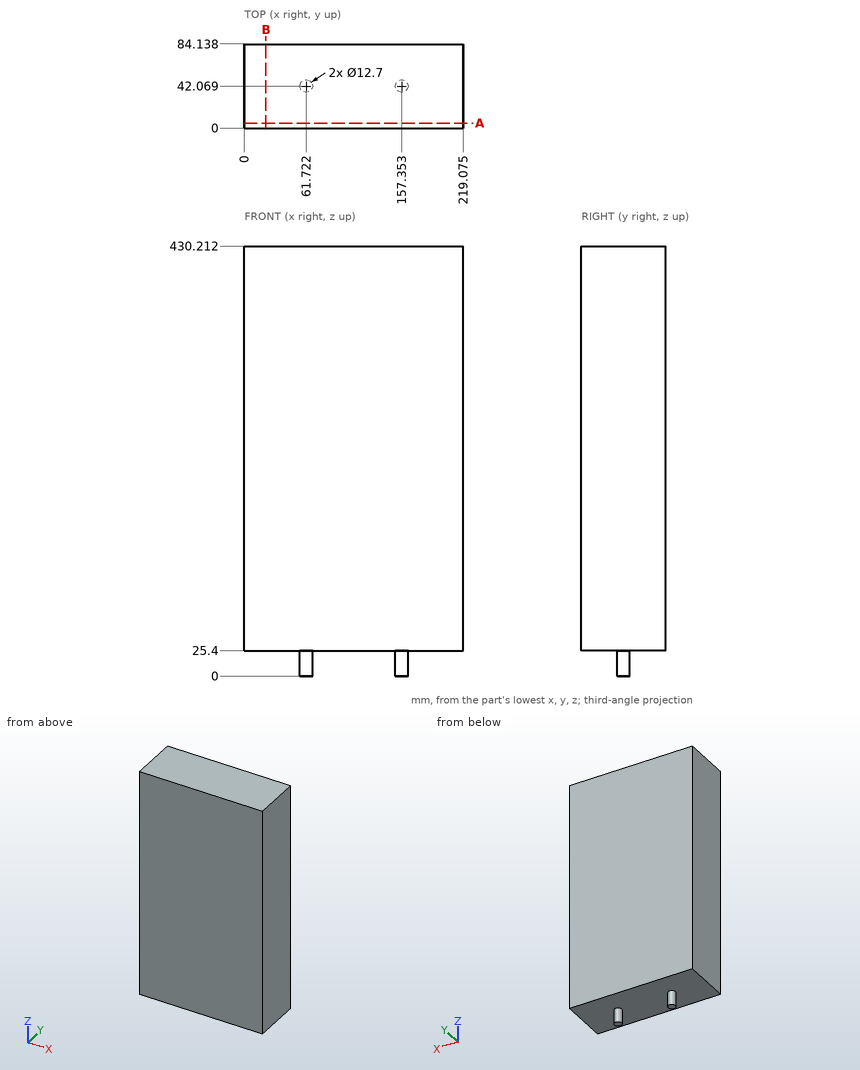
Geometry: see drawing. Coordinates: mm, zero at the bounding-box minimum. Give positions to 0.01 mm unless a question says otherwise; leave off trailing zeros. Write each loop counter-clockwise with the first axis right and the second up, starting at its lowest first coordinate (ties: lowest second). Pieces come first, ordered by that corner, then holes. Notation, with made-up numbers: (-14, 61.25) -> (24, 61.25) arc R5 cw to (24, 66.25) -> close; hole circle Ø8 at (11, -12.5). An arc over 180 degrees is marked (long way). Use one line per item in the form item = value. Start each with the question number.
1) Pin query (flat end, axial travel): pin 1 (6 mm diameter, centred on x = 138, y = 46.5, fed in from -Z). Return the tip coordinate at first contact, or that it passes through.
2) Ray query, probe 1 along Z at (x, y) = (87, 11). Return the intervals inside material, ascending. Write a range as from..to.
3) Section query A-A on y = 5. Return the cut outline in (x, z) (1 decimal), then the cut area to 3 significant figures.
4) Section query B-B on x = 21.5. Return the cut outline in (y, z), then the cut area to 3 significant figures.
Outcome:
q1.pin_1 = 25.4
q2.probe_1 = 25.4..430.21
q3.outline = (0, 25.4) -> (219.1, 25.4) -> (219.1, 430.2) -> (0, 430.2) -> close
q3.area = 88,700 mm^2
q4.outline = (0, 25.4) -> (84.14, 25.4) -> (84.14, 430.21) -> (0, 430.21) -> close
q4.area = 34,100 mm^2
